The listing builds one solid part. Answer for the finished solid, in the listing's coordinates (mm). A direction names the side the tool comes from. Round coordinates to 2 decimals unless told otherwise and drop trailing zeros. Write each loop counter-clockwise with the first axis right and the second up, starting at its lowest first coordinate (ties: lowest second). Pieces come first, ordered by that corner, then holes.
(1) For faces 1 (the face through (-1, -7, -28.5)), 2 (the face through (-34, -4.5, 34)), 3 (the face through (-17.75, -2, -41)), 4 (the face through (33, -1, -24)), 5 (the face through (29, -2, 34.5)), determine the directions among +Z, -Z, +X, -X, +Y, -Y from which every point of the face is accessible in a straight line to the end or side of a thin tool.
(2) A cutting plane is placed at D-D, the plane x = 8.5. Give the vertices of the cut face in (y, z), and give its area (3 significant figures).
(3) A cutting plane is placed at B-B, the plane z = -1. Give the vertices of the cut face in (x, y), and give its area (3 significant figures).
(4) The mould has two halves that part along X. Classify faces 6 (the face through (47.5, -2, -39)), 7 (the face through (12.5, -2, -39)), 8 (the face through (44.14, -6.51, -27.6)), 9 (the face through (-46.64, -2.22, 46.6)): +X half, -X half, draft (parallel to the pull), parting line (faces both ways), or undercut.
(5) Each of these flat-tipped pins is pushed along its axis until it touches: pin 1 Ø1 at (x, z) = (15.5, -41) entering from +Y; pin 2 Ø2 at (x, z) = (-27, 2.5) entering from -Y; pin 3 Ø2 at (y, z) = (-3, 42.5) entering from +X; pin 4 Ø2 at (y, z) = (-2.5, 41) entering from -X. Where does it stop, or does it pass through?
(6) A cutting plane is placed at C-C, the plane z = -14. Give the number of separate pieces and of enclosed holes in the cut face, and give its area (3 significant figures).
(7) A cutting plane is placed at A-A, the plane x = -21. Give the vertices of the cut face in (y, z), and give its area (3 significant figures).
(8) Find the intervals of material crossed by probe 1 along X at (y, z) = (-2.5, 33.8); probe 2 along Z at (x, y) = (43.5, -1.95); probe 3 along Z at (x, y) = (35, -1.25), in increasing order.
from build123d import *

# Parameters (mm, degrees)
SKETCH_1_R          = 1.5
SKETCH_1_R_2        = 0.8
EXTRUDE_1_DEPTH     = 9.6
CUT_EXTRUDE_START   = -5.1
CUT_EXTRUDE_1_DEPTH = 5.1
SKETCH_3_W          = 90
SKETCH_3_H          = 57
CUT_EXTRUDE_2_DEPTH = 7.1
FILLET_1_R          = 3
FILLET_2_R          = 1
SKETCH_13_W         = 12
SKETCH_13_H         = 12
CUT_EXTRUDE_3_DEPTH = 73.118652234


with BuildPart() as part:
    # 草图1 → 凸台-拉伸1 (new body)
    with BuildSketch(Plane(origin=(0, 0, 0), x_dir=(1, 0, 0), z_dir=(0, 1, 0))):
        with BuildLine():
            Line((-47.5, 23), (-47.5, -23))
            ThreePointArc((-47.5, -23), (-48.085786438, -24.414213562), (-49.5, -25))
            Line((-49.5, -25), (-50.8, -25))
            ThreePointArc((-50.8, -25), (-53.8, -28), (-50.8, -31))
            Line((-50.8, -31), (-49.5, -31))
            ThreePointArc((-49.5, -31), (-48.085786438, -31.585786438), (-47.5, -33))
            Line((-47.5, -33), (-47.5, -44.5))
            ThreePointArc((-47.5, -44.5), (-46.621320344, -46.621320344), (-44.5, -47.5))
            Line((-44.5, -47.5), (-41.25, -47.5))
            Line((-41.25, -47.5), (-41.25, -34.5))
            Line((-41.25, -34.5), (-17.75, -34.5))
            Line((-17.75, -34.5), (-17.75, -47.5))
            Line((-17.75, -47.5), (-15.5, -47.5))
            ThreePointArc((-15.5, -47.5), (-13.378679656, -46.621320344), (-12.5, -44.5))
            Line((-12.5, -44.5), (-12.5, -33))
            ThreePointArc((-12.5, -33), (-11.914213562, -31.585786438), (-10.5, -31))
            Line((-10.5, -31), (-5, -31))
            ThreePointArc((-5, -31), (-3.585786438, -31.585786438), (-3, -33))
            Line((-3, -33), (-3, -33.8))
            ThreePointArc((-3, -33.8), (0, -36.8), (3, -33.8))
            Line((3, -33.8), (3, -33))
            ThreePointArc((3, -33), (3.585786438, -31.585786438), (5, -31))
            Line((5, -31), (10.5, -31))
            ThreePointArc((10.5, -31), (11.914213562, -31.585786438), (12.5, -33))
            Line((12.5, -33), (12.5, -44.5))
            ThreePointArc((12.5, -44.5), (13.378679656, -46.621320344), (15.5, -47.5))
            Line((15.5, -47.5), (17.75, -47.5))
            Line((17.75, -47.5), (17.75, -34.5))
            Line((17.75, -34.5), (41.25, -34.5))
            Line((41.25, -34.5), (41.25, -47.5))
            Line((41.25, -47.5), (44.5, -47.5))
            ThreePointArc((44.5, -47.5), (46.621320344, -46.621320344), (47.5, -44.5))
            Line((47.5, -44.5), (47.5, -33))
            ThreePointArc((47.5, -33), (48.085786438, -31.585786438), (49.5, -31))
            Line((49.5, -31), (50.8, -31))
            ThreePointArc((50.8, -31), (53.8, -28), (50.8, -25))
            Line((50.8, -25), (49.5, -25))
            ThreePointArc((49.5, -25), (48.085786438, -24.414213562), (47.5, -23))
            Line((47.5, -23), (47.5, 23))
            ThreePointArc((47.5, 23), (48.085786438, 24.414213562), (49.5, 25))
            Line((49.5, 25), (50.8, 25))
            ThreePointArc((50.8, 25), (53.8, 28), (50.8, 31))
            Line((50.8, 31), (49.5, 31))
            ThreePointArc((49.5, 31), (48.085786438, 31.585786438), (47.5, 33))
            Line((47.5, 33), (47.5, 44.5))
            ThreePointArc((47.5, 44.5), (46.621320344, 46.621320344), (44.5, 47.5))
            Line((44.5, 47.5), (41.25, 47.5))
            Line((41.25, 47.5), (41.25, 34.5))
            Line((41.25, 34.5), (17.75, 34.5))
            Line((17.75, 34.5), (17.75, 47.5))
            Line((17.75, 47.5), (15.5, 47.5))
            ThreePointArc((15.5, 47.5), (13.378679656, 46.621320344), (12.5, 44.5))
            Line((12.5, 44.5), (12.5, 33))
            ThreePointArc((12.5, 33), (11.914213562, 31.585786438), (10.5, 31))
            Line((10.5, 31), (5, 31))
            ThreePointArc((5, 31), (3.585786438, 31.585786438), (3, 33))
            Line((3, 33), (3, 33.8))
            ThreePointArc((3, 33.8), (0, 36.8), (-3, 33.8))
            Line((-3, 33.8), (-3, 33))
            ThreePointArc((-3, 33), (-3.585786438, 31.585786438), (-5, 31))
            Line((-5, 31), (-10.5, 31))
            ThreePointArc((-10.5, 31), (-11.914213562, 31.585786438), (-12.5, 33))
            Line((-12.5, 33), (-12.5, 44.5))
            ThreePointArc((-12.5, 44.5), (-13.378679656, 46.621320344), (-15.5, 47.5))
            Line((-15.5, 47.5), (-17.75, 47.5))
            Line((-17.75, 47.5), (-17.75, 34.5))
            Line((-17.75, 34.5), (-41.25, 34.5))
            Line((-41.25, 34.5), (-41.25, 47.5))
            Line((-41.25, 47.5), (-44.5, 47.5))
            ThreePointArc((-44.5, 47.5), (-46.621320344, 46.621320344), (-47.5, 44.5))
            Line((-47.5, 44.5), (-47.5, 33))
            ThreePointArc((-47.5, 33), (-48.085786438, 31.585786438), (-49.5, 31))
            Line((-49.5, 31), (-50.8, 31))
            ThreePointArc((-50.8, 31), (-53.8, 28), (-50.8, 25))
            Line((-50.8, 25), (-49.5, 25))
            ThreePointArc((-49.5, 25), (-48.085786438, 24.414213562), (-47.5, 23))
        make_face()
        with Locations(Location((-50.8, 28, 0), (0, 0, 270))):
            Circle(SKETCH_1_R, mode=Mode.SUBTRACT)
        with Locations(Location((50.8, 28, 0), (0, 0, 90))):
            Circle(SKETCH_1_R, mode=Mode.SUBTRACT)
        with Locations(Location((50.8, -28, 0), (0, 0, 270))):
            Circle(SKETCH_1_R, mode=Mode.SUBTRACT)
        with Locations(Location((-50.8, -28, 0), (0, 0, 90))):
            Circle(SKETCH_1_R, mode=Mode.SUBTRACT)
        with Locations(Location((0, 33.8, 0), (0, 0, 270))):
            Circle(SKETCH_1_R, mode=Mode.SUBTRACT)
        with Locations(Location((0, -33.8, 0), (0, 0, 90))):
            Circle(SKETCH_1_R, mode=Mode.SUBTRACT)
        with Locations(Location((43.5, 41, 0), (0, 0, 270))):
            Circle(SKETCH_1_R_2, mode=Mode.SUBTRACT)
        with Locations(Location((15.5, 41, 0), (0, 0, 90))):
            Circle(SKETCH_1_R_2, mode=Mode.SUBTRACT)
        with Locations(Location((43.5, -41, 0), (0, 0, 90))):
            Circle(SKETCH_1_R_2, mode=Mode.SUBTRACT)
        with Locations(Location((15.5, -41, 0), (0, 0, 270))):
            Circle(SKETCH_1_R_2, mode=Mode.SUBTRACT)
        with Locations(Location((-15.5, -41, 0), (0, 0, 90))):
            Circle(SKETCH_1_R_2, mode=Mode.SUBTRACT)
        with Locations(Location((-43.5, -41, 0), (0, 0, 270))):
            Circle(SKETCH_1_R_2, mode=Mode.SUBTRACT)
        with Locations(Location((-43.5, 41, 0), (0, 0, 90))):
            Circle(SKETCH_1_R_2, mode=Mode.SUBTRACT)
        with Locations(Location((-15.5, 41, 0), (0, 0, 270))):
            Circle(SKETCH_1_R_2, mode=Mode.SUBTRACT)
    extrude(amount=-EXTRUDE_1_DEPTH)

    # 草图2 → 切除-拉伸1 (cut)
    with BuildSketch(Plane.XZ.offset(9.6).offset(CUT_EXTRUDE_START)):
        with BuildLine():
            Line((63.557901373, 31), (5, 31))
            ThreePointArc((5, 31), (3.585786438, 31.585786438), (3, 33))
            Line((3, 33), (3, 33.8))
            ThreePointArc((3, 33.8), (0, 36.8), (-3, 33.8))
            Line((-3, 33.8), (-3, 33))
            ThreePointArc((-3, 33), (-3.585786438, 31.585786438), (-5, 31))
            Line((-5, 31), (-73.010332056, 31))
            Line((-73.010332056, 31), (-73.010332056, 53.694218021))
            Line((-73.010332056, 53.694218021), (63.557901373, 53.694218021))
            Line((63.557901373, 53.694218021), (63.557901373, 31))
        make_face()
        with BuildLine():
            Line((63.557901373, -31), (63.557901373, -53.694218021))
            Line((63.557901373, -53.694218021), (-73.010332056, -53.694218021))
            Line((-73.010332056, -53.694218021), (-73.010332056, -31))
            Line((-73.010332056, -31), (-5, -31))
            ThreePointArc((-5, -31), (-3.585786438, -31.585786438), (-3, -33))
            Line((-3, -33), (-3, -33.8))
            ThreePointArc((-3, -33.8), (0, -36.8), (3, -33.8))
            Line((3, -33.8), (3, -33))
            ThreePointArc((3, -33), (3.585786438, -31.585786438), (5, -31))
            Line((5, -31), (63.557901373, -31))
        make_face()
    extrude(amount=CUT_EXTRUDE_1_DEPTH, mode=Mode.SUBTRACT)

    # 草图3 → 切除-拉伸2 (cut)
    with BuildSketch(Plane.XZ.offset(9.6)):
        Rectangle(SKETCH_3_W, SKETCH_3_H)
    extrude(amount=-CUT_EXTRUDE_2_DEPTH, mode=Mode.SUBTRACT)

    # 圆角1
    fillet_1_edges = [part.edges().sort_by_distance(p)[0] for p in [
        (45, -6.05, 28.5),
        (45, -6.05, -28.5),
        (-45, -6.05, -28.5),
        (-45, -6.05, 28.5),
    ]]
    fillet(fillet_1_edges, radius=FILLET_1_R)

    # 圆角2
    fillet_2_edges = [part.edges().sort_by_distance(p)[0] for p in [
        (0, -2.5, -28.5),
        (-45, -2.5, 0),
        (45, -2.5, 0),
        (0, -2.5, 28.5),
        (44.121320344, -2.5, 27.621320344),
        (44.121320344, -2.5, -27.621320344),
        (-44.121320344, -2.5, 27.621320344),
        (-44.121320344, -2.5, -27.621320344),
    ]]
    fillet(fillet_2_edges, radius=FILLET_2_R)

    # 草图13 → 切除-拉伸3 (cut, through all)
    with BuildSketch(Plane.XZ.offset(2.5)):
        with Locations((-33, 18)):
            Rectangle(SKETCH_13_W, SKETCH_13_H)
        with Locations((-16.6, 18)):
            Rectangle(SKETCH_13_W, SKETCH_13_H)
        with Locations((-0.2, 18)):
            Rectangle(SKETCH_13_W, SKETCH_13_H)
        with Locations((16.2, 18)):
            Rectangle(SKETCH_13_W, SKETCH_13_H)
        with Locations((32.6, 18)):
            Rectangle(SKETCH_13_W, SKETCH_13_H)
        with Locations((-16.6, 0)):
            Rectangle(SKETCH_13_W, SKETCH_13_H)
        with Locations((-0.2, 0)):
            Rectangle(SKETCH_13_W, SKETCH_13_H)
        with Locations((16.2, 0)):
            Rectangle(SKETCH_13_W, SKETCH_13_H)
        with Locations((-16.6, -18)):
            Rectangle(SKETCH_13_W, SKETCH_13_H)
        with Locations((-0.2, -18)):
            Rectangle(SKETCH_13_W, SKETCH_13_H)
        with Locations((16.2, -18)):
            Rectangle(SKETCH_13_W, SKETCH_13_H)
        with Locations((32.6, -18)):
            Rectangle(SKETCH_13_W, SKETCH_13_H)
        with Locations((-33, 0)):
            Rectangle(SKETCH_13_W, SKETCH_13_H)
        with Locations((-33, -18)):
            Rectangle(SKETCH_13_W, SKETCH_13_H)
    extrude(amount=-CUT_EXTRUDE_3_DEPTH, mode=Mode.SUBTRACT)


solid = part.part
Solutions:
1. face 1: -Y
1. face 2: +Z, -X, -Y
1. face 3: -Z, +Y, -Y
1. face 4: +Y, -Y
1. face 5: +Z, +Y, -Y
2. outline: (-9.6, -31) - (0, -31) - (0, 31) - (-9.6, 31) - (-9.6, 28.5) - (-3.5, 28.5) arc R1 cw to (-2.5, 27.5) - (-2.5, -27.5) arc R1 cw to (-3.5, -28.5) - (-9.6, -28.5) - close
2. area: 191 mm2
3. outline: (-47.5, -9.6) - (-45, -9.6) - (-45, -3.5) arc R1 cw to (-44, -2.5) - (-39, -2.5) - (-39, 0) - (-47.5, 0) - close; (-27, -2.5) - (-22.6, -2.5) - (-22.6, 0) - (-27, 0) - close; (-10.6, -2.5) - (-6.2, -2.5) - (-6.2, 0) - (-10.6, 0) - close; (5.8, -2.5) - (10.2, -2.5) - (10.2, 0) - (5.8, 0) - close; (22.2, -2.5) - (44, -2.5) arc R1 cw to (45, -3.5) - (45, -9.6) - (47.5, -9.6) - (47.5, 0) - (22.2, 0) - close
3. area: 153 mm2
4. face 6: +X half
4. face 7: undercut
4. face 8: undercut
4. face 9: -X half
5. pin 1: passes through
5. pin 2: stops at y = -2.5
5. pin 3: stops at x = 47.5
5. pin 4: stops at x = -47.5
6. separate pieces: 6
6. enclosed holes: 0
6. area: 123 mm2
7. outline: (-9.6, -31) - (-4.5, -31) - (-4.5, -34.5) - (0, -34.5) - (0, -24) - (-2.5, -24) - (-2.5, -27.5) arc R1 cw to (-3.5, -28.5) - (-9.6, -28.5) - close; (-9.6, 28.5) - (-3.5, 28.5) arc R1 cw to (-2.5, 27.5) - (-2.5, 24) - (0, 24) - (0, 34.5) - (-4.5, 34.5) - (-4.5, 31) - (-9.6, 31) - close; (-2.5, -12) - (0, -12) - (0, -6) - (-2.5, -6) - close; (-2.5, 6) - (0, 6) - (0, 12) - (-2.5, 12) - close
7. area: 132 mm2
8. probe 1: x = -47.5 to -12.5, -3 to -1.5, 1.5 to 3, 12.5 to 47.5
8. probe 2: z = -47.5 to -41.8, -40.2 to 40.2, 41.8 to 47.5
8. probe 3: z = -34.5 to -24, -12 to 12, 24 to 34.5
